The model under review builds one solid part; all positions refer to its coordinate system, in mm. Round coordinates to 2 decimals unless told otherwise and drop trailing zeros. Order: outer loops, then holes, each group sorted by start corner. A loop starts at its lowest first (then second) coordinate and runs counter-clockwise, first axis right, second up. Notation, with made-up numbers: M 6,40 L 37,40 A20 ccw 37,77 Z; hole C -32,49 d9. An arc over 180 degrees is marked long. Answer as a JSON object with one key per item and string values. Group by question number.
1. Add section C-C on y = -0.4. State the section outline as (x, z) points, and give its area (3 significant figures).
2. Add section A-A on x = 0. State the section outline as (y, z) points, and give its area (3 significant figures).
3. Add section B-B on z = 1. State the section outline as (x, y) points, and give its area (3 significant figures).
4. Clearance check with flat-ended pins moving along their axes: P1, Ø2.5, axis at x = 0, y = -0.4, coming from the -Z side (3 decimals); P2, Ø1, axis at y = 11, z = 2, coming from the -X side; P3, Ø1, axis at y = -5.5, z = 2.5, coming from the -X side. State where each tip first meets the part, or that it passes through.
5. Mouldability with a two-part tool opening along Y and no side actions: class faces 1 (the face through (96, 0, 1)), 2 (the face through (-1, -4, 3)), 3 (the face through (-53.048, -0.301, 1.521)) as released by +Y, released by -Y, zero draft, split by the parting line, or undercut.
6. Add section D-D on y = 8.5. State the section outline as (x, z) points.
7. To check wall thickness, follow probe 1 along X at (y, z) = (-0.4, 2.2); probe 2 along Y at (x, z) = (-50.8, 1.4); probe 3 along X at (y, z) = (-13.5, 2.15). State the ranges of each line that lie inside material, in increasing order. Write a range as [from, to].
Autodesk Inventor part; units mm, degrees
ref_plane "YZ Plane" through (0, 0, 0) normal (1, 0, 0) x (0, 1, 0)
ref_plane "XZ Plane" through (0, 0, 0) normal (0, 1, 0) x (-1, 0, 0)
ref_plane "XY Plane" through (0, 0, 0) normal (0, 0, 1) x (1, 0, 0)
sketch "Sketch1" plane through (0, 0, 0) normal (0, 0, 1) x (1, 0, 0)
  line L0 (-79, 0) -> (79, 0) construction
  line L1 (-79, -17) -> (79, -17)
  line L2 (79, 17) -> (-79, 17)
  arc A0 (-79, 17) -> (-79, -17) centre (-79, 0) ccw
  arc A1 (79, -17) -> (79, 17) centre (79, 0) ccw
  point P0 (0, 0)
  dimension "d0" = 79
  dimension "d1" = 34
extrude "Extrusion1" add sketch "Sketch1" along normal blind 3
sketch "Sketch2" plane through (0, 0, 3) normal (0, 0, 1) x (1, 0, 0)
  line L0 (63.5, 11.5) -> (-63.5, 11.5)
  line L1 (-63.5, 11.5) -> (-63.5, -11.5)
  line L2 (-63.5, -11.5) -> (63.5, -11.5)
  line L3 (63.5, -11.5) -> (63.5, 11.5)
  line L4 (63.5, 11.5) -> (-63.5, -11.5) construction
  line L5 (-63.5, 11.5) -> (63.5, -11.5) construction
  line L6 (-63.5, 0) -> (63.5, 0)
  circle A0 centre (-50.8, -0.4) radius 2.25
  circle A1 centre (50.8, -0.4) radius 2.25
  circle A2 centre (0, -0.4) radius 2.25
  point P0 (0, 0)
  dimension "d4" = 23
  dimension "d5" = 4.5
  dimension "d6" = 4.5
  dimension "d7" = 4.5
extrude "Extrusion2" cut sketch "Sketch2" against normal through all contours A1 L6 | L6 A1 | A0 L6 | L6 A0 | A2 L6 | L6 A2
properties part number "AMR_Handle_Flap"
Recorded:
{
 "1": {"outline": "M -96,0 L -53.05,0 L -53.05,3 L -96,3 Z; M -48.55,0 L -2.25,0 L -2.25,3 L -48.55,3 Z; M 2.25,0 L 48.55,0 L 48.55,3 L 2.25,3 Z; M 53.05,0 L 96,0 L 96,3 L 53.05,3 Z", "area": "535 mm²"},
 "2": {"outline": "M -17,0 L -2.65,0 L -2.65,3 L -17,3 Z; M 1.85,0 L 17,0 L 17,3 L 1.85,3 Z", "area": "88.5 mm²"},
 "3": {"outline": "M -79,-17 L 79,-17 A17 ccw 79,17 L -79,17 A17 ccw Z; hole C -50.8,-0.4 d4.5; hole C 0,-0.4 d4.5; hole C 50.8,-0.4 d4.5", "area": "6,230 mm²"},
 "4": {"P1": "passes through", "P2": "stops at x = -92.37", "P3": "stops at x = -95.25"},
 "5": {"face 1": "split by the parting line", "face 2": "zero draft", "face 3": "undercut"},
 "6": {"outline": "M -93.72,0 L 93.72,0 L 93.72,3 L -93.72,3 Z"},
 "7": {"probe 1": "x = [-96, -53.05], [-48.55, -2.25], [2.25, 48.55], [53.05, 96]", "probe 2": "y = [-17, -2.65], [1.85, 17]", "probe 3": "x = [-89.33, 89.33]"}
}
